Model file for the job. Use its own axes, mm. A direction names the side the tool comes from. Round coordinates to 2 decimals unless told otherwise and drop trailing zeros. Loops run counter-clockwise (first coordinate to the right, second up) from the corner with the lowest first, then second, coordinate; pieces in that order, holes last.
from build123d import *

# Parameters (mm, degrees)
SKETCH1_W               = 700
SKETCH1_H               = 500
BOSS_EXTRUDE1_DEPTH     = 50
SKETCH2_W               = 560
SKETCH2_H               = 420
SKETCH2_W_2             = 540
SKETCH2_H_2             = 400
EXTRUDE_THIN1_DEPTH     = 250
CUT_EXTRUDE5_DEPTH      = 71
CUT_EXTRUDE5_DEPTH_BACK = 631
SKETCH4_R               = 80
CUT_EXTRUDE6_DEPTH      = 51


with BuildPart() as part:
    # Sketch1 → Boss-Extrude1 (new body)
    with BuildSketch(Plane.XY):
        Rectangle(SKETCH1_W, SKETCH1_H)
    extrude(amount=BOSS_EXTRUDE1_DEPTH)

    # Sketch2 → Extrude-Thin1 (add)
    with BuildSketch(Plane.XY.offset(50)):
        Rectangle(SKETCH2_W, SKETCH2_H)
        Rectangle(SKETCH2_W_2, SKETCH2_H_2, mode=Mode.SUBTRACT)
    extrude(amount=EXTRUDE_THIN1_DEPTH)

    # Sketch3 → Cut-Extrude5 (cut, two sides)
    with BuildSketch(Plane.ZY.offset(280)) as cut_extrude5_sk:
        Polygon((300, 210), (175, 210), (300, -210), align=None)
    extrude(amount=CUT_EXTRUDE5_DEPTH, mode=Mode.SUBTRACT)
    extrude(cut_extrude5_sk.sketch, amount=-CUT_EXTRUDE5_DEPTH_BACK, mode=Mode.SUBTRACT)

    # Sketch4 → Cut-Extrude6 (cut, through all)
    with BuildSketch(Plane.XY.offset(50)):
        with Locations((0, -62)):
            Circle(SKETCH4_R)
    extrude(amount=-CUT_EXTRUDE6_DEPTH, mode=Mode.SUBTRACT)


solid = part.part
Q1. Slice it at C-C on z = 271.5. Give the cut face in (x, y).
Q2. Flat gauge pins, fed straight in: P1, Ø4, axis at x = -10, y = 56, coming from the -Z side; P2, Ø1, axis at y = 196.5, z = 136.5, coming from the -X side; P3, Ø8, axis at x = -270.5, y = 108.5, coming from the +Z side; P4, Ø12, axis at x = 164, y = 82.5, coming from the +Z side. Where does each tip first touch, or does it go through?
Q3. Tool access for faces 1 (the face through (-270, -3, 144)), 2 (the face through (-4, -210, 173)), 3 (the face through (-4, 210, 112)), 4 (the face through (-5, 59, 0)), 5 (the face through (-280, -3, 145)): list every direction of +Z, -Z, +X, -X, +Y, -Y with a clear straight run to the whole face (end or side of a thin tool).
Q4. Slice it at B-B on y = -62. Give the cut face in (x, z).
Q5. Slice it at A-A on x = 0. Give the cut face in (y, z).
Q6. Probe line 1 (X direction, y = -64.5, z = 139); line 2 (Y direction, x = -151, z = 146); line 3 (Y direction, x = 0, z = 35.5). List the from-to ranges inside material, lowest first.
Q7. Slice it at D-D on x = 157.5. Give the cut face in (y, z), plus the area to 4 significant figures.
Q8. Pull direction X, two halves, no side cores. Call faces 6 (the face through (-350, -3, 25)), 7 (the face through (280, -3, 145)), 8 (the face through (-270.94, 0.98, 237.21)), 9 (the face through (270, -3, 144)): pulls with the +X half, pulls with the -X half, needs draft (parallel to the pull), parting line crosses it, or undercut.
Reply:
1. outline: (-280, -210) - (280, -210) - (280, -114.24) - (270, -114.24) - (270, -200) - (-270, -200) - (-270, -114.24) - (-280, -114.24) - close
2. P1: stops at z = 0
2. P2: stops at x = -280
2. P3: stops at z = 206.4
2. P4: stops at z = 50
3. face 1: +Z
3. face 2: +Z, +X, -X, -Y
3. face 3: +Z, +X, -X, +Y
3. face 4: -Z, +X, -X, +Y, -Y
3. face 5: +Z, -X, +Y, -Y
4. outline: (-350, 0) - (-80, 0) - (-80, 50) - (-270, 50) - (-270, 255.95) - (-280, 255.95) - (-280, 50) - (-350, 50) - close; (80, 0) - (350, 0) - (350, 50) - (280, 50) - (280, 255.95) - (270, 255.95) - (270, 50) - (80, 50) - close
5. outline: (-250, 0) - (-142, 0) - (-142, 50) - (-200, 50) - (-200, 297.02) - (-210, 300) - (-210, 50) - (-250, 50) - close; (18, 0) - (250, 0) - (250, 50) - (210, 50) - (210, 175) - (200, 177.98) - (200, 50) - (18, 50) - close
6. line 1: x = -280 to -270, 270 to 280
6. line 2: y = -210 to -200, 200 to 210
6. line 3: y = -250 to -142, 18 to 250
7. outline: (-250, 0) - (250, 0) - (250, 50) - (210, 50) - (210, 175) - (200, 177.98) - (200, 50) - (-200, 50) - (-200, 297.02) - (-210, 300) - (-210, 50) - (-250, 50) - close
7. area: 28,750 mm2
8. face 6: pulls with the -X half
8. face 7: pulls with the +X half
8. face 8: needs draft
8. face 9: undercut
